```python
from build123d import *

# Parameters (mm, degrees)
SKETCH1_R           = 5
BOSS_EXTRUDE1_DEPTH = 20
SKETCH2_R           = 5
SKETCH2_R_2         = 3.98
CUT_EXTRUDE2_DEPTH  = 8
SKETCH8_R           = 5
BOSS_EXTRUDE2_DEPTH = 20
BOSS_EXTRUDE3_START = -31.5
BOSS_EXTRUDE3_DEPTH = 31.5
BOSS_EXTRUDE4_START = -31.5
BOSS_EXTRUDE4_DEPTH = 31.5
SKETCH12_R          = 7.5
SKETCH12_R_2        = 6
CUT_EXTRUDE3_DEPTH  = 31.5
CUT_EXTRUDE4_DEPTH  = 55.083269132
FILLET1_R           = 10
BOSS_EXTRUDE5_START = 13
SKETCH17_R          = 3.98
BOSS_EXTRUDE5_DEPTH = 13
CUT_EXTRUDE5_DEPTH  = 46.417762115
SKETCH19_R          = 5
SKETCH19_R_2        = 3.98
CUT_EXTRUDE6_DEPTH  = 0.5
SKETCH20_R          = 3.98
SKETCH20_R_2        = 3.8
CUT_EXTRUDE7_DEPTH  = 21.5
FILLET2_R           = 1.5


with BuildPart() as part:
    # Sketch1 → Boss-Extrude1 (new body)
    with BuildSketch(Plane.XY):
        Circle(SKETCH1_R)
    extrude(amount=BOSS_EXTRUDE1_DEPTH)

    # Sketch2 → Cut-Extrude2 (cut)
    with BuildSketch(Plane(origin=(0, 0, 0), x_dir=(-1, 0, 0), z_dir=(0, 0, -1))):
        Circle(SKETCH2_R)
        Circle(SKETCH2_R_2, mode=Mode.SUBTRACT)
    extrude(amount=-CUT_EXTRUDE2_DEPTH, mode=Mode.SUBTRACT)

    # Sketch8 → Boss-Extrude2 (add)
    with BuildSketch(Plane.XY.offset(20)):
        with Locations(Location((0, 0, 0), (0, 0, 180))):
            Circle(SKETCH8_R)
    extrude(amount=BOSS_EXTRUDE2_DEPTH)

    # Sketch9 → Boss-Extrude3 (add)
    with BuildSketch(Plane.XY.offset(40).offset(BOSS_EXTRUDE3_START)):
        with BuildLine():
            Line((0, 5), (35, 5))
            Line((35, 5), (35, -5))
            Line((35, -5), (0, -5))
            ThreePointArc((0, -5), (5, 0), (0, 5))
        make_face()
    extrude(amount=BOSS_EXTRUDE3_DEPTH)

    # Sketch10 → Boss-Extrude4 (add)
    with BuildSketch(Plane.XY.offset(40).offset(BOSS_EXTRUDE4_START)):
        with BuildLine():
            ThreePointArc((0, -5), (-5, 0), (0, 5))
            Line((0, 5), (-15, 5))
            Line((-15, 5), (-15, -5))
            Line((-15, -5), (0, -5))
        make_face()
    extrude(amount=BOSS_EXTRUDE4_DEPTH)

    # Sketch12 → Cut-Extrude3 (cut)
    with BuildSketch(Plane(origin=(0, 5, 0), x_dir=(1, 0, 0), z_dir=(0, 1, 0))):
        with Locations(Location((0, -21.5, 0), (0, 0, 270))):
            Circle(SKETCH12_R)
        with Locations(Location((17.579426131, -25.368304137, 0), (0, 0, 270))):
            Circle(SKETCH12_R_2)
    extrude(amount=-CUT_EXTRUDE3_DEPTH, mode=Mode.SUBTRACT)

    # Sketch14 → Cut-Extrude4 (cut, through all)
    with BuildSketch(Plane(origin=(0, 5, 0), x_dir=(1, 0, 0), z_dir=(0, 1, 0))):
        Polygon((-15, -40), (35, -40), (35, -37.368304137), (35, -8.5), (10, -8.5), (27.579426131, -18.251873125), (27.579426131, -35.368304137), (-15, -32.5), align=None)
    extrude(amount=-CUT_EXTRUDE4_DEPTH, mode=Mode.SUBTRACT)

    # Fillet1
    fillet1_edges = [part.edges().sort_by_distance(p)[0] for p in [
        (-15, 0, 8.5),
        (27.579426131, 0, 18.251873125),
        (10, 0, 8.5),
        (-15, 0, 32.5),
        (27.579426131, 0, 35.368304137),
    ]]
    fillet(fillet1_edges, radius=FILLET1_R - 0.0001)  # a hair under: the kernel refuses the full size

    # Sketch17 → Boss-Extrude5 (add)
    with BuildSketch(Plane(origin=(0, 0, 0), x_dir=(-1, 0, 0), z_dir=(0, 0, -1)).offset(BOSS_EXTRUDE5_START)):
        Circle(SKETCH17_R)
    extrude(amount=-BOSS_EXTRUDE5_DEPTH)

    # Sketch18 → Cut-Extrude5 (cut, through all)
    with BuildSketch(Plane(origin=(0, 5, 0), x_dir=(1, 0, 0), z_dir=(0, 1, 0))):
        with BuildLine():
            Line((-1.6, 11.5), (1.6, 11.5))
            ThreePointArc((1.6, 11.5), (1.882842712, 11.382842712), (2, 11.1))
            Line((2, 11.1), (2, 9.9))
            ThreePointArc((2, 9.9), (1.882842712, 9.617157288), (1.6, 9.5))
            Line((1.6, 9.5), (-1.6, 9.5))
            ThreePointArc((-1.6, 9.5), (-1.882842712, 9.617157288), (-2, 9.9))
            Line((-2, 9.9), (-2, 11.1))
            ThreePointArc((-2, 11.1), (-1.882842712, 11.382842712), (-1.6, 11.5))
        make_face()
    extrude(amount=-CUT_EXTRUDE5_DEPTH, mode=Mode.SUBTRACT)

    # Sketch19 → Cut-Extrude6 (cut)
    with BuildSketch(Plane(origin=(0, 0, 8), x_dir=(-1, 0, 0), z_dir=(0, 0, -1))):
        Circle(SKETCH19_R)
        Circle(SKETCH19_R_2, mode=Mode.SUBTRACT)
    extrude(amount=-CUT_EXTRUDE6_DEPTH, mode=Mode.SUBTRACT)

    # Sketch20 → Cut-Extrude7 (cut)
    with BuildSketch(Plane(origin=(0, 0, -13), x_dir=(-1, 0, 0), z_dir=(0, 0, -1))):
        Circle(SKETCH20_R)
        Circle(SKETCH20_R_2, mode=Mode.SUBTRACT)
    extrude(amount=-CUT_EXTRUDE7_DEPTH, mode=Mode.SUBTRACT)

    # Fillet2
    fillet2_edges = [part.edges().sort_by_distance(p)[0] for p in [
        (3.8, 0, 8.5),
    ]]
    fillet(fillet2_edges, radius=FILLET2_R)


solid = part.part
```
Geometry check sheet. Reference: the model listing, model coordinates, mm. A direction names the side the tool comes from. Round coordinates to 2 decimals unless told otherwise and drop trailing zeros. Order: outer loops, then holes, each group sorted by start corner. A loop starts at its lowest first (then second) coordinate and runs counter-clockwise, first axis right, second up. Notation, with made-up numbers: (-14, 60) - (23, 60) arc R25 cw to (23, 80) - close; hole circle Ø8 at (56.25, 66.25). An arc over 180 degrees is marked (long way). Use a Markdown table: item, result. Add a question column.
1) Mould release check, pull along X, two halves, no side actions. Record for faces 5 (the cylindrical face through (9.952, -0.07, 8.828)), 6 (the flat face through (5.8, 0.1, 33.9)), 7 (the flat face through (-2, 0, -10.5)): released by +X, released by -X, zero draft, split by the parting line, or undercut.
2) Thickness scan on line 1 along X through (y, z) = (-0.5, 21.5); line 2 along X through (y, z) = (0.25, 6.5); line 3 along Z through (x, y) = (2.5, 3). Record the ranges inside material, lowest first.
3) Section check B-B (x = 0). Count the separate pieces of the cut face and the enclosed holes in it, then the cut area to 3 significant figures.
4) Set-up check for faces 1 (the flat face through (-4, 4, 8.5)), 2 (the flat face through (0, 0, -9.5)), 3 (the flat face through (-4, -4, 8.5)), 4 (the cylindrical face through (0.49, 3.77, -3.12)): record each of +Z, -Z, +X, -X, +Y, -Y from which the full face is reachable in a straight line by a thin tool's end or side.
5) Section check C-C (x = -12). Record the cut outline in (y, z), then the cut area to 3 significant figures.
6) Gauge pin test, flat ends, axial feed: P1, Ø4, axis at y = -1, z = -3.5, coming from the +X side; P2, Ø1.5, axis at x = 16, y = 0.5, coming from the +Z side; P3, Ø2, axis at x = 20.5, y = 0.5, coming from the -Z side; P4, Ø7, axis at x = 17.58, z = 25.37, coming from the +Y side. Record the tip position at first contact, or that the pin passes through.
7) Section check A-A (z = 21.5). Record the cut outline in (x, y), then the cut area to 3 significant figures.
Established:
| question | item | result |
|---|---|---|
| 1 | face 5 | released by +X |
| 1 | face 6 | released by -X |
| 1 | face 7 | undercut |
| 2 | line 1 | -15 to -7.5, 7.5 to 12.99, 22.17 to 27.22 |
| 2 | line 2 | -3.79 to 3.79 |
| 2 | line 3 | 7.55 to 14.43, 28.57 to 33.68 |
| 3 | separate pieces | 3 |
| 3 | enclosed holes | 0 |
| 3 | area | 249 mm2 |
| 4 | face 1 | -Z, -X, +Y |
| 4 | face 2 | +Y, -Y |
| 4 | face 3 | -Z, -X, -Y |
| 4 | face 4 | -Z |
| 5 | outline | (-5, 11.36) - (5, 11.36) - (5, 30.29) - (-5, 30.29) - close |
| 5 | area | 189 mm2 |
| 6 | P1 | x = 3.8 |
| 6 | P2 | z = 34.64 |
| 6 | P3 | z = 13.77 |
| 6 | P4 | through |
| 7 | outline | (-15, -5) - (-7.5, -5) - (-7.5, 5) - (-15, 5) - close; (7.5, -5) - (12.99, -5) - (12.99, 5) - (7.5, 5) - close; (22.17, -5) - (27.22, -5) - (27.22, 5) - (22.17, 5) - close |
| 7 | area | 181 mm2 |
